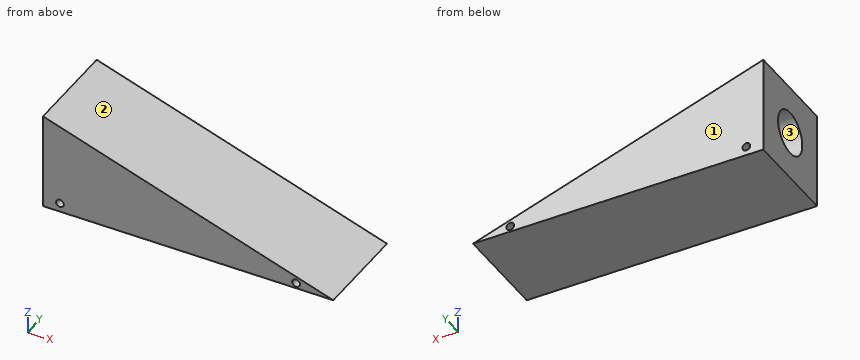
```python
from build123d import *

# Parameters (mm, degrees)
F1_DEPTH = 25.4
F2_R     = 5.715
F3_DEPTH = 17.78
F4_R     = 1.016
F5_DEPTH = 25.4
F6_R     = 1.016
F7_DEPTH = 25.4


with BuildPart() as f1:
    # F0 (on Front) → F1 (new body)
    with BuildSketch(Plane.XZ):
        Polygon((-76.2, 0), (0, 0), (-76.2, 25.4), align=None)
    extrude(amount=F1_DEPTH)

    # F2 (on face) → F3 (cut)
    with BuildSketch(Plane(origin=(-76.2, 0, 0), x_dir=(0, -1, 0), z_dir=(-1, 0, 0))):
        with Locations((12.7, 12.7)):
            Circle(F2_R)
    extrude(amount=-F3_DEPTH, mode=Mode.SUBTRACT)

    # F4 (on face) → F5 (cut)
    with BuildSketch(Plane.XZ.offset(25.4)):
        with Locations((-71.755275, 2.325441)):
            Circle(F4_R)
    extrude(amount=-F5_DEPTH, mode=Mode.SUBTRACT)

    # F6 (on face) → F7 (cut)
    with BuildSketch(Plane.XZ.offset(25.4)):
        with Locations((-9.774557, 1.460582)):
            Circle(F6_R)
    extrude(amount=-F7_DEPTH, mode=Mode.SUBTRACT)


solid = f1.part
```
CAD build for the part. Positions are in the model's coordinates, mm. Face numbers are marked on the shaded views. Give positions to 0.01 mm unless a question says otherwise; leave off trailing zeros. Order: outer loops, then holes, each group sorted by start corner. A loop starts at its lowest first (then second) coordinate and runs counter-clockwise, first axis right, second up.
(1) Saw through at B-B, the plane z = 12.7. Give the cut face in (x, y) (3 decimals), then the cut area to 3 significant figures.
(2) Mould opens along Y. For the marked faces 1, 2 and 3 say: released by +Y, released by -Y, zero draft, split by the parting line, or undercut.
(3) Flat gauge pins, fed straight in: pin 1 (3 mm diameter, centred on x = -66, y = -5.5, fed in from +Z); pin 2 (1.6 mm diameter, centred on x = -71.76, z = 2.33, fed in from -Y); pin 3 (4 mm diameter, centred on x = -43.5, y = -16.5, fed in from +Z); pin 4 (5.5 mm diameter, centred on y = -15.5, z = 12, fed in from -X). Where does each tip first touch, or does it go through?
(4) Saw through at D-D, the plane y = -8.75. Give the cut face in (x, z), then the cut area to 3 significant figures.
(5) Saw through at A-A, the plane y = -12.7. Give the cut face in (x, z) (3 decimals).
(6) Saw through at C-C, the plane x = -68. Give the cut face in (y, z) (3 decimals), then the cut area to 3 significant figures.
(7) Drill centre lines: L1, parallel to Z at x = -67, y = -12.7 (3 decimals); L2, parallel to Z at x = -62, y = -19.5; L3, parallel to Z at x = -6.5, y = -21.5. Where is each one in solid material? Low to high.
Results found:
1. outline: (-76.2, -25.4) - (-38.1, -25.4) - (-38.1, 0) - (-76.2, 0) - (-76.2, -6.985) - (-58.42, -6.985) - (-58.42, -18.415) - (-76.2, -18.415) - close
1. area: 765 mm2
2. face 1: released by +Y
2. face 2: zero draft
2. face 3: undercut
3. pin 1: stops at z = 22.5
3. pin 2: passes through
3. pin 3: stops at z = 15.17
3. pin 4: stops at x = -58.42
4. outline: (-76.2, 0) - (0, 0) - (-76.2, 25.4) - (-76.2, 16.83) - (-58.42, 16.83) - (-58.42, 8.57) - (-76.2, 8.57) - close; hole circle Ø2.03 at (-71.76, 2.33); hole circle Ø2.03 at (-9.77, 1.46)
4. area: 814 mm2
5. outline: (-76.2, 0) - (0, 0) - (-76.2, 25.4) - (-76.2, 18.415) - (-58.42, 18.415) - (-58.42, 6.985) - (-76.2, 6.985) - close; hole circle Ø2.032 at (-71.755, 2.325); hole circle Ø2.032 at (-9.775, 1.461)
6. outline: (-25.4, 0) - (0, 0) - (0, 22.667) - (-25.4, 22.667) - close; hole circle Ø11.43 at (-12.7, 12.7)
6. area: 473 mm2
7. L1: z = 0 to 6.985, 18.415 to 22.333
7. L2: z = 0 to 20.67
7. L3: z = 0 to 2.17
